Check sheet for the modelled part. Datum: model origin and axes. Units: mm. A direction names the side the tool comes from. Round coordinates to 2 decimals unless told otherwise and drop trailing zeros. Write each loop counter-clockwise with the first axis right and the second up, starting at its lowest first coordinate (ties: lowest second). Pieces come first, ordered by that corner, then holes.
Item 1: Depth check by flat-ended pin: pin 1 (4 mm diameter, centred on x = 6.5, y = 0.5, fed in from +Z); pin 2 (3 mm diameter, centred on x = 1, y = 2, fed in from -Z); pin 3 (1 mm diameter, centred on x = -7.5, z = 2.5, fed in from +Y); pin 4 (6 mm diameter, centred on x = -6, y = 1, fed in from +Z). Enter the tip coordinate at first touch or a pass-through.
Item 2: Section check C-C, the plane x = 0. Record the cut outline in (y, z).
Item 3: Material ranges on line 1 along Y through (x, z) = (0, 0.6); line 2 along X through (y, z) = (0, 0.3); line 3 along Z through (x, y) = (2.25, 2), recorded low to high.
Item 4: Section check D-D, the plane y = 2. Record the cut outline in (x, z).
Item 5: Section check A-A, the plane z = 1.5. Record the cut outline in (x, y), plus the area to 3 significant figures.
Item 6: Section check B-B, the plane z = 0.4. Record the cut outline in (x, y), plus the area to 3 significant figures.
Item 7: Set-up check for faces 1 (the flat face through (2.5, 5, 1)), 2 (the flat face through (-5, -4, 0.6)), 3 (the flat face through (-5, 4, 0.6)): record each of +Z, -Z, +X, -X, +Y, -Y from which the full face is reachable in a straight line by a thin tool's end or side.
from build123d import *

# Parameters (mm, degrees)
PAD_DEPTH    = 0.6
PAD001_DEPTH = 0.7
PAD002_DEPTH = 1.4
SKETCH003_R  = 0.4
PAD003_DEPTH = 1
PAD004_DEPTH = 2.5
SKETCH005_R  = 5
POCKET_DEPTH = 1


with BuildPart() as part:
    # Sketch → Pad (new body)
    with BuildSketch(Plane.XY):
        with BuildLine():
            ThreePointArc((-7.987387, 2.907171), (-8.5, 0), (-7.987387, -2.907171))
            Line((-7.496671, -2.792834), (-7.987387, -2.907171))
            ThreePointArc((-7.496671, -2.792834), (-6.789372, -4.231363), (-5.809475, -5.5))
            Line((5.809475, -5.5), (-5.809475, -5.5))
            ThreePointArc((5.809475, -5.5), (6.789372, -4.231363), (7.496671, -2.792834))
            Line((7.496671, -2.792834), (7.987387, -2.907171))
            ThreePointArc((7.987387, -2.907171), (8.5, 0), (7.987387, 2.907171))
            Line((7.496671, 2.792834), (7.987387, 2.907171))
            ThreePointArc((7.496671, 2.792834), (6.789372, 4.231363), (5.809475, 5.5))
            Line((-5.809475, 5.5), (5.809475, 5.5))
            ThreePointArc((-5.809475, 5.5), (-6.789372, 4.231363), (-7.496671, 2.792834))
            Line((-7.987387, 2.907171), (-7.496671, 2.792834))
        make_face()
    extrude(amount=PAD_DEPTH)

    # Sketch001 (on Face14 of Pad) → Pad001 (join)
    with BuildSketch(Plane.XY.offset(0.6)):
        with BuildLine():
            ThreePointArc((-7.987387, 2.907171), (-8.5, 0), (-7.987387, -2.907171))
            Line((-3.037451, -1.105543), (-7.987387, -2.907171))
            ThreePointArc((-3.037451, 1.105543), (-3.232388, 0), (-3.037451, -1.105543))
            Line((-7.987387, 2.907171), (-3.037451, 1.105543))
        make_face()
        with BuildLine():
            ThreePointArc((7.987387, -2.907171), (8.5, 0), (7.987387, 2.907171))
            Line((3.166555, 1.05855), (7.987387, 2.907171))
            ThreePointArc((3.137447, -1.141937), (3.33851, -0.044161), (3.166555, 1.05855))
            Line((7.987387, -2.907171), (3.137447, -1.141937))
        make_face()
    extrude(amount=PAD001_DEPTH)

    # Sketch002 (on Face5 of Pad001) → Pad002 (join)
    with BuildSketch(Plane.XY.offset(0.6)):
        with BuildLine():
            Line((-2.5, 5.5), (-2.5, 4.616546))
            ThreePointArc((-2.5, 4.616546), (-5.25, 0), (-2.5, -4.616546))
            Line((-2.5, -5.5), (-2.5, -4.616546))
            Line((2.5, -5.5), (-2.5, -5.5))
            Line((2.5, -5.5), (2.5, -4.616546))
            ThreePointArc((2.5, -4.616546), (5.25, 0), (2.5, 4.616546))
            Line((2.5, 5.5), (2.5, 4.616546))
            Line((2.5, 5.5), (-2.5, 5.5))
        make_face()
    extrude(amount=PAD002_DEPTH)

    # Sketch003 → Pad003 (join)
    with BuildSketch(Plane.XY):
        with Locations((-8.1, 0)):
            Circle(SKETCH003_R)
        with Locations((8.1, 0)):
            Circle(SKETCH003_R)
    extrude(amount=-PAD003_DEPTH)

    # Sketch004 (on Face37 of Pad003) → Pad004 (join)
    with BuildSketch(Plane.XY.offset(1.3)):
        with BuildLine():
            Line((-8.4, 1.4), (-7.2, 1.4))
            Line((-7.2, 1.4), (-7.2, -1.4))
            Line((-7.2, -1.4), (-8.4, -1.4))
            ThreePointArc((-8.4, 1.4), (-8.515868, 0), (-8.4, -1.4))
        make_face()
    extrude(amount=PAD004_DEPTH)

    # Sketch005 (on Face4 of Pad004) → Pocket (cut)
    with BuildSketch(Plane(origin=(0, 0, 0), x_dir=(1, 0, 0), z_dir=(0, 0, -1))):
        Circle(SKETCH005_R)
    extrude(amount=-POCKET_DEPTH, mode=Mode.SUBTRACT)


solid = part.part
Values found:
1. pin 1: stops at z = 2
1. pin 2: stops at z = 1
1. pin 3: stops at y = 1.4
1. pin 4: stops at z = 3.8
2. outline: (-5.5, 0) - (-5, 0) - (-5, 1) - (5, 1) - (5, 0) - (5.5, 0) - (5.5, 2) - (-5.5, 2) - close
3. line 1: y = -5.5 to -5, 5 to 5.5
3. line 2: x = -8.5 to -5, 5 to 8.5
3. line 3: z = 1 to 2
4. outline: (-8.26, 0) - (-4.58, 0) - (-4.58, 1) - (4.58, 1) - (4.58, 0) - (8.26, 0) - (8.26, 1.3) - (5.62, 1.3) - (5.62, 0.6) - (4.85, 0.6) - (4.85, 2) - (-4.85, 2) - (-4.85, 0.6) - (-5.49, 0.6) - (-5.49, 1.3) - (-8.26, 1.3) - close
5. outline: (-8.4, -1.4) - (-7.2, -1.4) - (-7.2, 1.4) - (-8.4, 1.4) arc R8.52 ccw to start; (-2.5, -5.5) - (2.5, -5.5) - (2.5, -4.62) arc R5.25 ccw to (2.5, 4.62) - (2.5, 5.5) - (-2.5, 5.5) - (-2.5, 4.62) arc R5.25 ccw to (-2.5, -4.62) - close
5. area: 94.7 mm2
6. outline: (-7.99, -2.91) - (-7.5, -2.79) arc R8 ccw to (-5.81, -5.5) - (5.81, -5.5) arc R8 ccw to (7.5, -2.79) - (7.99, -2.91) arc R8.5 ccw to (7.99, 2.91) - (7.5, 2.79) arc R8 ccw to (5.81, 5.5) - (-5.81, 5.5) arc R8 ccw to (-7.5, 2.79) - (-7.99, 2.91) arc R8.5 ccw to start; hole circle Ø10 at (0, 0)
6. area: 88.2 mm2
7. face 1: +Z, +X, +Y
7. face 2: +Z, -Y
7. face 3: +Z, +Y
